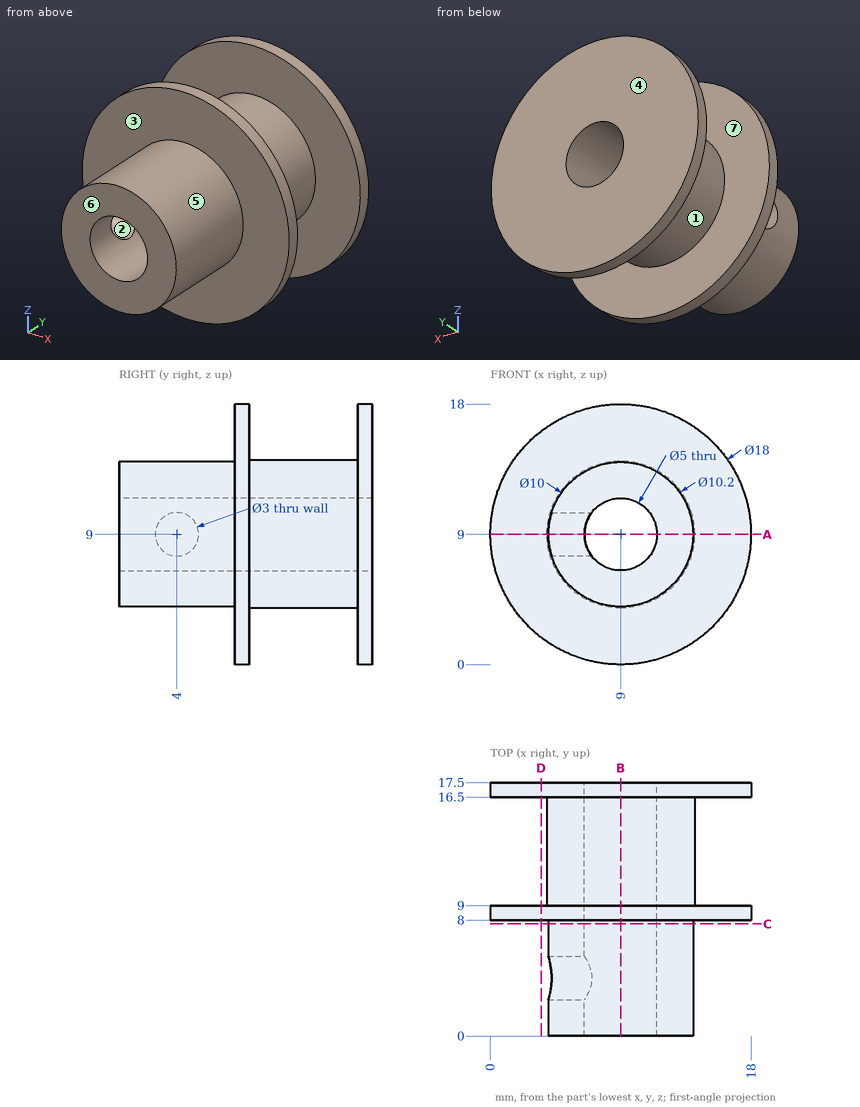
Study the drawing (mm; zero at the part's minimum x, y, z) and answer. A direction names the side the tool comes from. Round coordinates to 2 decimals unless told otherwise and drop trailing zeros. Order: outer loops, then holes, each group sorted by start corner. A loop starts at its lowest first (then second) coordinate and runs counter-clockwise, first axis right, second up. Notation, with made-up numbers: (15, 32) - (66, 32) arc R17 cw to (66, 36) - close; hole circle Ø3 at (33.25, 29). An arc over 180 degrees is marked (long way). Use one line per item in the form item = value. Start each with the question number.
(1) The part is cut by section B-B (x = 9). Give the vertices of the cut face in (y, z), then the cut area to 3 significant figures.
(2) The part is cut by section A-A (z = 9). Give the vertices of the cut face in (x, y).
(3) The part is cut by section D-D (x = 3.5). Give the vertices of the cut face in (y, z), then the cut area to 3 significant figures.
(4) For the marked faces 5, 6 and 7, determine the directions among +Z, -Z, +X, -X, +Y, -Y from which every point of the face is accessible in a straight line to the end or side of a thin tool.
(5) The part is cut by section C-C (y = 7.75). Give the vertices of the cut face in (x, z).
(6) Find the intervals of material crossed by line 1 along Y through (x, z) = (5.7, 9); line 2 along Y through (x, z) = (14.75, 4.5); line 3 along X through (y, z) = (5, 9), in increasing order. Write a range as from..to.
(7) Flat-ended cylindrical pins translate along their axes: pin 1 Ø2.5 at (y, z) = (4, 9) entering from -X; pin 2 Ø8 at (y, z) = (2.5, 10) entering from +X; pin 3 Ø1 at (y, z) = (10.5, 7) entering from -X. Find the tip coordinate at first contact, or state that the pin passes through.
(8) Determine the mould class of the marked faces 1, 2, 3 and 4 for opening direction Y: +Y half, -Y half, draft (parallel to the pull), parting line (faces both ways), or undercut.
Checked values:
q1.outline = (0, 4) - (8, 4) - (8, 0) - (9, 0) - (9, 3.9) - (16.5, 3.9) - (16.5, 0) - (17.5, 0) - (17.5, 6.5) - (0, 6.5) - close; (0, 11.5) - (17.5, 11.5) - (17.5, 18) - (16.5, 18) - (16.5, 14.1) - (9, 14.1) - (9, 18) - (8, 18) - (8, 14) - (0, 14) - close
q1.area = 105 mm^2
q2.outline = (0, 8) - (4, 8) - (4, 5.5) - (6.5, 5.5) - (6.5, 17.5) - (0, 17.5) - (0, 16.5) - (3.9, 16.5) - (3.9, 9) - (0, 9) - close; (4, 0) - (6.5, 0) - (6.5, 2.5) - (4, 2.5) - close; (11.5, 0) - (14, 0) - (14, 8) - (18, 8) - (18, 9) - (14.1, 9) - (14.1, 16.5) - (18, 16.5) - (18, 17.5) - (11.5, 17.5) - close
q3.outline = (8, 1.88) - (9, 1.88) - (9, 16.12) - (8, 16.12) - close; (16.5, 1.88) - (17.5, 1.88) - (17.5, 16.12) - (16.5, 16.12) - close
q3.area = 28.5 mm^2
q4.face_5 = -Y
q4.face_6 = +Z, -Z, +X, -X, -Y
q4.face_7 = none
q5.outline = circle Ø10 at (9, 9); hole circle Ø5 at (9, 9)
q6.line_1 = 0..2.5, 5.5..17.5
q6.line_2 = 8..9, 16.5..17.5
q6.line_3 = 11.5..14
q7.pin_1 = 11.17
q7.pin_2 = 14
q7.pin_3 = 4.13
q8.face_1 = undercut
q8.face_2 = undercut
q8.face_3 = -Y half
q8.face_4 = +Y half
